```python
from build123d import *

# Parameters (mm, degrees)
F0_W     = 50.8
F0_H     = 25.4
F0_R     = 12.7
F1_DEPTH = 3.175


with BuildPart() as f1:
    # F0 (on Top) → F1 (new body)
    with BuildSketch(Plane.XY):
        with BuildLine():
            Line((-50.8, 25.4), (-12.7, 25.4))
            ThreePointArc((-12.7, 25.4), (-3.719744, 21.680256), (0, 12.7))
            ThreePointArc((0, 12.7), (3.719744, 3.719744), (12.7, 0))
            Line((12.7, 0), (139.7, 0))
            ThreePointArc((139.7, 0), (148.680256, 3.719744), (152.4, 12.7))
            ThreePointArc((152.4, 12.7), (156.119744, 21.680256), (165.1, 25.4))
            Line((165.1, 25.4), (177.8, 25.4))
            ThreePointArc((177.8, 25.4), (186.780256, 29.119744), (190.5, 38.1))
            Line((190.5, 38.1), (190.5, 139.7))
            ThreePointArc((190.5, 139.7), (186.780256, 148.680256), (177.8, 152.4))
            Line((177.8, 152.4), (165.1, 152.4))
            ThreePointArc((165.1, 152.4), (156.119744, 156.119744), (152.4, 165.1))
            ThreePointArc((152.4, 165.1), (148.680256, 174.080256), (139.7, 177.8))
            Line((139.7, 177.8), (12.7, 177.8))
            ThreePointArc((12.7, 177.8), (3.719744, 174.080256), (0, 165.1))
            ThreePointArc((0, 165.1), (-3.719744, 156.119744), (-12.7, 152.4))
            Line((-12.7, 152.4), (-50.8, 152.4))
            ThreePointArc((-50.8, 152.4), (-59.780256, 148.680256), (-63.5, 139.7))
            Line((-63.5, 139.7), (-63.5, 38.1))
            ThreePointArc((-63.5, 38.1), (-59.780256, 29.119744), (-50.8, 25.4))
        make_face()
        with BuildLine():
            Line((-12.7, 38.1), (-50.8, 38.1))
            Line((-50.8, 38.1), (-50.8, 63.5))
            Line((-50.8, 63.5), (0, 63.5))
            Line((0, 63.5), (0, 50.8))
            ThreePointArc((0, 50.8), (-3.719744, 41.819744), (-12.7, 38.1))
        make_face(mode=Mode.SUBTRACT)
        with Locations((-25.4, 88.9)):
            Rectangle(F0_W, F0_H, mode=Mode.SUBTRACT)
        with BuildLine():
            Line((12.7, 38.1), (12.7, 88.9))
            Line((12.7, 88.9), (139.7, 88.9))
            Line((139.7, 88.9), (139.7, 38.1))
            ThreePointArc((139.7, 38.1), (135.980256, 29.119744), (127, 25.4))
            Line((127, 25.4), (25.4, 25.4))
            ThreePointArc((25.4, 25.4), (16.419744, 29.119744), (12.7, 38.1))
        make_face(mode=Mode.SUBTRACT)
        with Locations((165.1, 50.8)):
            Circle(F0_R, mode=Mode.SUBTRACT)
        with Locations((165.1, 88.9)):
            Circle(F0_R, mode=Mode.SUBTRACT)
        with BuildLine():
            Line((-50.8, 114.3), (-50.8, 139.7))
            Line((-50.8, 139.7), (0, 139.7))
            Line((0, 139.7), (0, 127))
            ThreePointArc((0, 127), (-3.719744, 118.019744), (-12.7, 114.3))
            Line((-12.7, 114.3), (-50.8, 114.3))
        make_face(mode=Mode.SUBTRACT)
        with Locations((165.1, 127)):
            Circle(F0_R, mode=Mode.SUBTRACT)
        with BuildLine():
            ThreePointArc((12.7, 139.7), (16.419744, 148.680256), (25.4, 152.4))
            Line((25.4, 152.4), (127, 152.4))
            ThreePointArc((127, 152.4), (135.980256, 148.680256), (139.7, 139.7))
            Line((139.7, 139.7), (139.7, 120.65))
            Line((139.7, 120.65), (12.7, 120.65))
            Line((12.7, 120.65), (12.7, 139.7))
        make_face(mode=Mode.SUBTRACT)
    extrude(amount=F1_DEPTH)


solid = f1.part
```
Here's how the part is built. I have some questions about the finished solid (model axes, mm). A direction names the side the tool comes from. Coordinates: 2 decimals unless noted, no trailing zeros. Write each loop counter-clockwise with the first axis right and the second up, starting at its lowest first coordinate (ties: lowest second). Pieces come first, ordered by that corner, then holes. Notation, with made-up numbers: (-6.75, 23) - (46.25, 23) arc R21 ccw to (46.25, 58) - close; hole circle Ø6 at (15, 32). An arc over 180 degrees is marked (long way). One line per item, written item: value.
1) I need wall thicknesses on line 1 along Y through (x, z) = (165.1, 1.4); line 2 along Y through (x, z) = (83.5, 1.45); line 3 along X through (y, z) = (50.5, 0.35). Which ranges of each line are inside material? Lowest first, please.
Model answer:
line 1: y = 25.4 to 38.1, 63.5 to 76.2, 101.6 to 114.3, 139.7 to 152.4
line 2: y = 0 to 25.4, 88.9 to 120.65, 152.4 to 177.8
line 3: x = -63.5 to -50.8, 0 to 12.7, 139.7 to 152.4, 177.8 to 190.5
2) Suppose I cut it at C-C on y = 135.5. Write out the boundary of the cut face in (x, z) (3 decimals), and give its area (3 significant figures).
Model answer:
outline: (-63.5, 0) - (-50.8, 0) - (-50.8, 3.175) - (-63.5, 3.175) - close; (0, 0) - (12.7, 0) - (12.7, 3.175) - (0, 3.175) - close; (139.7, 0) - (155.664, 0) - (155.664, 3.175) - (139.7, 3.175) - close; (174.536, 0) - (190.5, 0) - (190.5, 3.175) - (174.536, 3.175) - close
area: 182 mm²
3) Suppose I cut it at A-A on y = 70. Write out the boundary of the cut face in (x, z) (3 decimals).
Model answer:
outline: (-63.5, 0) - (12.7, 0) - (12.7, 3.175) - (-63.5, 3.175) - close; (139.7, 0) - (190.5, 0) - (190.5, 3.175) - (139.7, 3.175) - close
4) Suppose I cut it at B-B on x = 113. Write out the boundary of the cut face in (y, z) (3 decimals), and give its area (3 significant figures).
Model answer:
outline: (0, 0) - (25.4, 0) - (25.4, 3.175) - (0, 3.175) - close; (88.9, 0) - (120.65, 0) - (120.65, 3.175) - (88.9, 3.175) - close; (152.4, 0) - (177.8, 0) - (177.8, 3.175) - (152.4, 3.175) - close
area: 262 mm²
5) On a 3-axis mill with a long thin cutter (end or side, diameter ignored), from which of +Z, -Z, +X, -X, +Y, -Y can I reach the whole of each face in a straight line? I mean faces 1 (the cylindrical face through (-59.68, 148.78, 1.57)), 2 (the cylindrical face through (16.32, 148.58, 1.57)). Say none if no direction works.
Model answer:
face 1: +Z, -Z, -X, +Y
face 2: +Z, -Z
6) Suppose I cut it at D-D on x = 170.5. Write out the boundary of the cut face in (y, z) (3 decimals).
Model answer:
outline: (25.4, 0) - (39.305, 0) - (39.305, 3.175) - (25.4, 3.175) - close; (62.295, 0) - (77.405, 0) - (77.405, 3.175) - (62.295, 3.175) - close; (100.395, 0) - (115.505, 0) - (115.505, 3.175) - (100.395, 3.175) - close; (138.495, 0) - (152.4, 0) - (152.4, 3.175) - (138.495, 3.175) - close
7) I'm going to push flat-ended pins straight in: P1, Ø1, axis at x = -18, z = 1, coming from the -Y side; P2, Ø1.6, axis at x = -26, z = 1, coming from the +Y side; P3, Ø10, axis at x = 29.5, y = 30.5, coming from the -Z side. Where does each tip first touch, or does it pass through?
Model answer:
P1: stops at y = 25.4
P2: stops at y = 152.4
P3: passes through
8) We'd pull the mould along X, two halves only. Please class faces 3 (the flat face through (62, 90, 0)), 4 (the cylindrical face through (162.35, 114.6, 1.57)), 5 (the cylindrical face through (-59.88, 29.22, 1.57)): pulls with the +X half, pulls with the -X half, needs draft (parallel to the pull), parting line crosses it, or undercut.
Model answer:
face 3: needs draft
face 4: undercut
face 5: pulls with the -X half
